Input: part model. Units: mm. Frame: model coordinates. Round coordinates to 2 decimals unless told otherwise and drop trailing zeros. Write each loop counter-clockwise with the first axis right and the second up, starting at its lowest first coordinate (ties: lowest second). Pieces come first, ordered by that corner, then holes. Notation, with made-up numbers: (62, 79.5) - (99, 79.5) arc R26 ccw to (99, 112.5) - close; hole circle Ø6 at (75, 11). An arc over 180 degrees is marked (long way). Use one line per item in the form item = value.
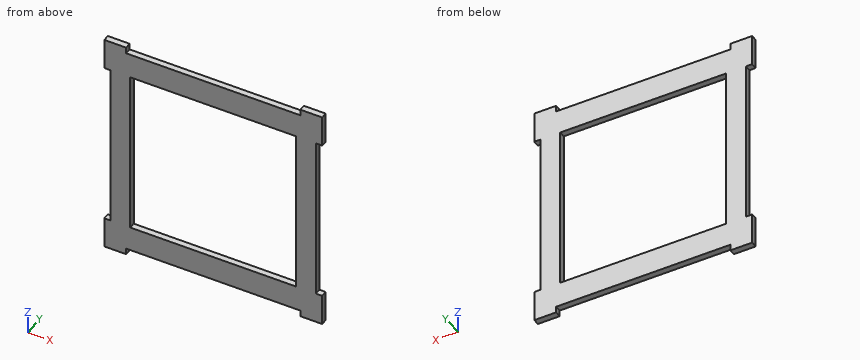
```python
from build123d import *

# Parameters (mm, degrees)
SKETCH2_W               = 109
SKETCH2_H               = 104
SKETCH2_W_2             = 80
SKETCH2_H_2             = 80
BOSS_EXTRUDE2_DEPTH     = 3
SKETCH3_W               = 12.5
SKETCH3_H               = 3
BOSS_EXTRUDE3_DEPTH     = 5
SKETCH4_W               = 5
SKETCH4_H               = 80
CUT_EXTRUDE1_DEPTH      = 5
SKETCH5_W               = 10.5
SKETCH5_H               = 2
CUT_EXTRUDE2_DEPTH      = 10
MIRROR5_COPY_1_SKETCH_W = 10.5
MIRROR5_COPY_1_SKETCH_H = 2
MIRROR5_COPY_1_DEPTH    = 10


with BuildPart() as part:
    # Sketch2 → Boss-Extrude2 (new body)
    with BuildSketch(Plane(origin=(0, 0, 0), x_dir=(1, 0, 0), z_dir=(0, 1, 0))):
        Rectangle(SKETCH2_W, SKETCH2_H)
        Rectangle(SKETCH2_W_2, SKETCH2_H_2, mode=Mode.SUBTRACT)
    extrude(amount=BOSS_EXTRUDE2_DEPTH)

    # Sketch3 → Boss-Extrude3 (add)
    with BuildSketch(Plane(origin=(0, 0, -52), x_dir=(-1, 0, 0), z_dir=(0, 0, -1))):
        with Locations((48.25, 1.5)):
            Rectangle(SKETCH3_W, SKETCH3_H)
    extrude(amount=BOSS_EXTRUDE3_DEPTH)

    # Mirror1: part across plane


with BuildPart() as part_1:
    add(part.part)
    add(part.part.mirror(Plane.XY))

    # Mirror2: part across plane


with BuildPart() as part_2:
    add(part_1.part)
    add(part_1.part.mirror(Plane(origin=(0, 0, 0), x_dir=(0, 0, 1), z_dir=(1, 0, 0))))

    # Sketch4 → Cut-Extrude1 (cut)
    with BuildSketch(Plane.XZ):
        with Locations((-52, 0)):
            Rectangle(SKETCH4_W, SKETCH4_H)
    cut_extrude1 = extrude(amount=-CUT_EXTRUDE1_DEPTH, mode=Mode.SUBTRACT)

    # Mirror3: Cut-Extrude1 across plane
    add(cut_extrude1.mirror(Plane(origin=(0, 0, 0), x_dir=(0, 0, 1), z_dir=(1, 0, 0))), mode=Mode.SUBTRACT)

    # Sketch5 → Cut-Extrude2 (cut)
    with BuildSketch(Plane.XZ):
        with Locations((47.25, -56)):
            Rectangle(SKETCH5_W, SKETCH5_H)
        Polygon((54.5, -57), (54.5, -40), (52.5, -40), (52.5, -55), (52.5, -57), align=None)
    cut_extrude2 = extrude(amount=-CUT_EXTRUDE2_DEPTH, mode=Mode.SUBTRACT)

    # Mirror4: Cut-Extrude2 across plane
    add(cut_extrude2.mirror(Plane(origin=(0, 0, 0), x_dir=(0, 0, 1), z_dir=(1, 0, 0))), mode=Mode.SUBTRACT)

    # Mirror5: Cut-Extrude2 across plane
    add(cut_extrude2.mirror(Plane.XY), mode=Mode.SUBTRACT)

    # Mirror5 copy 1 sketch → Mirror5 copy 1 (cut)
    with BuildSketch(Plane(origin=(0, 0, 0), x_dir=(-1, 0, 0), z_dir=(0, -1, 0))):
        with Locations((47.25, -56)):
            Rectangle(MIRROR5_COPY_1_SKETCH_W, MIRROR5_COPY_1_SKETCH_H)
        Polygon((54.5, -57), (54.5, -40), (52.5, -40), (52.5, -55), (52.5, -57), align=None)
    extrude(amount=-MIRROR5_COPY_1_DEPTH, mode=Mode.SUBTRACT)


solid = part_2.part
```
(1) Cut plane C-C on y = 2.4. Output: boundary loops of the cut face in (x, z), then the cut area to 3 significant figures.
Derived:
outline = (-52.5, -55) - (-42, -55) - (-42, -52) - (42, -52) - (42, -55) - (52.5, -55) - (52.5, -40) - (49.5, -40) - (49.5, 40) - (52.5, 40) - (52.5, 55) - (42, 55) - (42, 52) - (-42, 52) - (-42, 55) - (-52.5, 55) - (-52.5, 40) - (-49.5, 40) - (-49.5, -40) - (-52.5, -40) - close; hole (-40, -40) - (40, -40) - (40, 40) - (-40, 40) - close
area = 4,170 mm^2
(2) Cut plane A-A on z = 12. Output: boundary loops of the cut face in (x, y).
Derived:
outline = (-49.5, 0) - (-40, 0) - (-40, 3) - (-49.5, 3) - close; (40, 0) - (49.5, 0) - (49.5, 3) - (40, 3) - close
(3) Material intervals for L1, parallel to X at y = 1.45, z = -18; L2, parallel to Z at x = -3, y = 1.9; L3, parallel to Z at x = 40.5, y = 0.3, sorted ascending.
Derived:
L1 = -49.5 to -40, 40 to 49.5
L2 = -52 to -40, 40 to 52
L3 = -52 to 52
(4) First-contact query: pin 1 Ø1.5 at (x, y) = (12.5, 1) entering from -Z; pin 2 Ø1.5 at (x, y) = (19.5, 0.5) entering from +Z; pin 3 Ø4 at (x, z) = (3.5, -37) entering from -Y; pin 4 Ø8 at (x, z) = (-38.5, -1.5) entering from +Y. Flat tips, straight axial feed; report the tip coordinate or a pass-through.
Derived:
pin_1 = -52
pin_2 = 52
pin_3 = through
pin_4 = 3
(5) Cut plane B-B on x = 26. Output: boundary loops of the cut face in (y, z).
Derived:
outline = (0, -52) - (3, -52) - (3, -40) - (0, -40) - close; (0, 40) - (3, 40) - (3, 52) - (0, 52) - close
